```python
from build123d import *

# Parameters (mm, degrees)
SKETCH1_R           = 16
SKETCH1_R_2         = 9
SKETCH1_R_3         = 1.5
BOSS_EXTRUDE3_DEPTH = 13.5
SKETCH1_6_R         = 9
SKETCH1_6_R_2       = 7.5
BOSS_EXTRUDE4_DEPTH = 15.75
BOSS_EXTRUDE6_START = -31.5
SKETCH2_R           = 7.5
SKETCH2_R_2         = 2.75
BOSS_EXTRUDE6_DEPTH = 31.5


with BuildPart() as part:
    # Sketch1 → Boss-Extrude3 (new, symmetric)
    with BuildSketch(Plane.XY):
        Circle(SKETCH1_R)
        Circle(SKETCH1_R_2, mode=Mode.SUBTRACT)
        with Locations((-8.485281374, -8.485281374)):
            Circle(SKETCH1_R_3, mode=Mode.SUBTRACT)
        with Locations((8.485281374, -8.485281374)):
            Circle(SKETCH1_R_3, mode=Mode.SUBTRACT)
        with Locations((8.485281374, 8.485281374)):
            Circle(SKETCH1_R_3, mode=Mode.SUBTRACT)
        with Locations((-8.485281374, 8.485281374)):
            Circle(SKETCH1_R_3, mode=Mode.SUBTRACT)
    extrude(amount=BOSS_EXTRUDE3_DEPTH, both=True)

    # Sketch1<6> → Boss-Extrude4 (add, symmetric)
    with BuildSketch(Plane.XY):
        Circle(SKETCH1_6_R)
        Circle(SKETCH1_6_R_2, mode=Mode.SUBTRACT)
    extrude(amount=BOSS_EXTRUDE4_DEPTH, both=True)

    # Sketch2 → Boss-Extrude6 (add)
    # profile 1 of 3: a face of its own
    with BuildSketch(Plane.XY.offset(15.75).offset(BOSS_EXTRUDE6_START)):
        Circle(SKETCH2_R)
        Circle(SKETCH2_R_2, mode=Mode.SUBTRACT)
    # profile 2 of 3: a face of its own
    with BuildSketch(Plane.XY.offset(15.75).offset(BOSS_EXTRUDE6_START)):
        with BuildLine():
            ThreePointArc((2.121320344, 1.75), (0, 2.75), (-2.121320344, 1.75))
            Line((-2.121320344, 1.75), (2.121320344, 1.75))
        make_face()
    # profile 3 of 3: a face of its own
    with BuildSketch(Plane.XY.offset(15.75).offset(BOSS_EXTRUDE6_START)):
        with BuildLine():
            Line((2.121320344, -1.75), (-2.121320344, -1.75))
            ThreePointArc((-2.121320344, -1.75), (0, -2.75), (2.121320344, -1.75))
        make_face()
    extrude(amount=BOSS_EXTRUDE6_DEPTH)


solid = part.part
```
Check sheet for the modelled part. Datum: model origin and axes. Units: mm. A direction names the side the tool comes from. Round coordinates to 2 decimals unless told otherwise and drop trailing zeros. Order: outer loops, then holes, each group sorted by start corner. A loop starts at its lowest first (then second) coordinate and runs counter-clockwise, first axis right, second up. Notation, with made-up numbers: (-4.75, -29.5) - (1.25, -29.5) arc R15 cw to (1.25, -5.5) - close; hole circle Ø4 at (58.5, 80). An arc over 180 degrees is marked (long way). Answer as CSV lines item,"result". Start each with the question number.
1) Draft check along Y on faces 4 (the face through (9.29, 9.75, -0.19)), 5 (the face through (-2.75, 0.03, -0.22)), 6 (the face through (-1.172, 8.923, -14.609)), 7 (the face through (7, -7, 13.5)). Enter one of: +Y half, -Y half, draft (parallel to the pull), parting line (faces both ways), or undercut.
2) Tool access check on faces 1 (the face through (7, -7, -13.5)), 2 (the face through (-1.172, 8.923, 14.641)), 3 (the face through (2.75, -0.03, -0.22)). Record the directions out of +Z, -Z, +X, -X, +Y, -Y that give a thin tool (end or side, any length) a straight path to the whole face; none if there is none.
3) Section check A-A (x = 0). Record the cut outline in (y, z).
4) Depth check by flat-ended pin: pin 1 (2 mm diameter, centred on x = 6, z = -10.5, fed in from -Y); pin 2 (3 mm diameter, centred on y = -12, z = 8, fed in from +X); pin 3 (3.5 mm diameter, centred on x = -8.49, y = 8.49, fed in from -Z); pin 4 (2.5 mm diameter, centred on x = 8.49, y = -8.49, fed in from -Z). Enter the tip coordinate at first touch or a pass-through.
5) Section check B-B (y = 0). Record the cut outline in (x, z).
6) Scan lines: probe 1 along Y at (x, z) = (-0.5, -9.5); probe 2 along Y at (x, z) = (-7.5, 2.5); probe 3 along Y at (x, z) = (-8, -7). Record each from-to range of solid material in increasing order.
7) Section check D-D (y = -6.5). Record the cut outline in (x, z), then the cut area to 3 significant figures.
8) Section check C-C (z = -5.5). Record the cut outline in (x, y), then the cut area to 3 significant figures.
Determined:
1,face 4,"undercut"
1,face 5,"undercut"
1,face 6,"parting line"
1,face 7,"draft"
2,face 1,"-Z"
2,face 2,"+Z"
2,face 3,"+Z, -Z"
3,outline,"(-16, -13.5) - (-9, -13.5) - (-9, -15.75) - (-1.75, -15.75) - (-1.75, 15.75) - (-9, 15.75) - (-9, 13.5) - (-16, 13.5) - close; (1.75, -15.75) - (9, -15.75) - (9, -13.5) - (16, -13.5) - (16, 13.5) - (9, 13.5) - (9, 15.75) - (1.75, 15.75) - close"
4,pin 1,"y = -15.2"
4,pin 2,"x = 12.07"
4,pin 3,"z = -13.5"
4,pin 4,"through"
5,outline,"(-16, -13.5) - (-9, -13.5) - (-9, -15.75) - (-2.75, -15.75) - (-2.75, 15.75) - (-9, 15.75) - (-9, 13.5) - (-16, 13.5) - close; (2.75, -15.75) - (9, -15.75) - (9, -13.5) - (16, -13.5) - (16, 13.5) - (9, 13.5) - (9, 15.75) - (2.75, 15.75) - close"
6,probe 1,"-15.99 to -1.75, 1.75 to 15.99"
6,probe 2,"-14.13 to -9.62, -7.35 to 7.35, 9.62 to 14.13"
6,probe 3,"-13.86 to -9.9, -7.07 to 7.07, 9.9 to 13.86"
7,outline,"(-14.62, -13.5) - (-6.22, -13.5) - (-6.22, -15.75) - (6.22, -15.75) - (6.22, -13.5) - (14.62, -13.5) - (14.62, 13.5) - (6.22, 13.5) - (6.22, 15.75) - (-6.22, 15.75) - (-6.22, 13.5) - (-14.62, 13.5) - close"
7,area,"846 mm^2"
8,outline,"circle Ø32 at (0, 0); hole circle Ø3 at (-8.49, -8.49); hole circle Ø3 at (-8.49, 8.49); hole (-2.12, -1.75) - (2.12, -1.75) arc R2.75 ccw to (2.12, 1.75) - (-2.12, 1.75) arc R2.75 ccw to start; hole circle Ø3 at (8.49, -8.49); hole circle Ø3 at (8.49, 8.49)"
8,area,"758 mm^2"
